from build123d import *

# Parameters (mm, degrees)
EXTRUDE_1_DEPTH             = 30
HOLE_WIZARD_M31_D           = 3.4
HOLE_WIZARD_M31_CBORE_D     = 6.5
HOLE_WIZARD_M31_CBORE_DEPTH = 3


with BuildPart() as part:
    # Эскиз1 → Бобышка-Вытянуть1 (new body)
    with BuildSketch(Plane.XY):
        Polygon((-3, 0), (-11, 0), (-11, 8), (11, 8), (11, 0), (3, 0), (3, 3), (-3, 3), align=None)
    extrude(amount=EXTRUDE_1_DEPTH)

    # Цековка для винта с внутренним шестигранником M31 (through all)
    with Locations(Plane(origin=(0, 8, 0), x_dir=(1, 0, 0), z_dir=(0, 1, 0))):
        with Locations((-7, -4), (7, -4), (7, -26), (-7, -26)):
            CounterBoreHole(HOLE_WIZARD_M31_D / 2, HOLE_WIZARD_M31_CBORE_D / 2, HOLE_WIZARD_M31_CBORE_DEPTH)


solid = part.part
Can you work these out from the model? Positions are in its coordinate system, mm. A direction names the side the tool comes from. Round coordinates to 2 decimals unless told otherwise and drop trailing zeros. Write each loop counter-clockwise with the first axis right and the second up, starting at its lowest first coordinate (ties: lowest second). Pieces come first, ordered by that corner, then holes. Notation, with made-up numbers: M 52,55 L 60,55 A32 cw 60,88 Z; hole C -6,31.25 d10. An arc over 180 degrees is marked long. Use a Markdown table: item, result.
Item 1: If I drill on line 1 along X through (y, z) = (2.45, 26); line 2 along X through (y, z) = (6.5, 26); line 3 along Z through (x, y) = (-7, 3.15), over which ranges is the centre line in solid material (lowest first)? Write a range as [from, to].
Found:
| item | result |
|---|---|
| line 1 | x = [-11, -8.7], [-5.3, -3], [3, 5.3], [8.7, 11] |
| line 2 | x = [-11, -10.25], [-3.75, 3.75], [10.25, 11] |
| line 3 | z = [0, 2.3], [5.7, 24.3], [27.7, 30] |
Item 2: I want a section at D-D (z = 19). List the corners of the cut face in (x, y) for me, and give its area (3 significant figures).
Found:
| item | result |
|---|---|
| outline | M -11,0 L -3,0 L -3,3 L 3,3 L 3,0 L 11,0 L 11,8 L -11,8 Z |
| area | 158 mm2 |
Item 3: I want a section at B-B (x = 7). List the corners of the cut face in (y, z) for me.
Found:
| item | result |
|---|---|
| outline | M 0,0 L 8,0 L 8,0.75 L 5,0.75 L 5,2.3 L 0,2.3 Z; M 0,5.7 L 5,5.7 L 5,7.25 L 8,7.25 L 8,22.75 L 5,22.75 L 5,24.3 L 0,24.3 Z; M 0,27.7 L 5,27.7 L 5,29.25 L 8,29.25 L 8,30 L 0,30 Z |
Item 4: We'd pull the mould along Z, two halves only. Please class faces 1 (the face through (3, 1, 15)), 2 (the face through (0, 4, 0)), 3 (the face through (-10.247, 6.521, 3.857)): released by +Z, released by -Z, zero draft, split by the parting line, or undercut.
Found:
| item | result |
|---|---|
| face 1 | zero draft |
| face 2 | released by -Z |
| face 3 | undercut |
Item 5: I want a section at C-C (y = 7). List the corners of the cut face in (x, z) for me.
Found:
| item | result |
|---|---|
| outline | M -11,0 L 11,0 L 11,30 L -11,30 Z; hole C -7,4 d6.5; hole C -7,26 d6.5; hole C 7,4 d6.5; hole C 7,26 d6.5 |
Item 6: I want a section at A-A (z = 26). List the corners of the cut face in (x, y) for me.
Found:
| item | result |
|---|---|
| outline | M -11,0 L -8.7,0 L -8.7,5 L -10.25,5 L -10.25,8 L -11,8 Z; M -5.3,0 L -3,0 L -3,3 L 3,3 L 3,0 L 5.3,0 L 5.3,5 L 3.75,5 L 3.75,8 L -3.75,8 L -3.75,5 L -5.3,5 Z; M 8.7,0 L 11,0 L 11,8 L 10.25,8 L 10.25,5 L 8.7,5 Z |
Item 7: Which directions (+Z, -Z, +X, -X, +Y, -Y) give clear straight access to the entire face, cutting with the end or side of a thin tool? Please do faces 4 (the face through (8.4, 5, 27.4)), 5 (the face through (0, 8, 15)), 6 (the face through (-3, 2, 15)).
Found:
| item | result |
|---|---|
| face 4 | +Y |
| face 5 | +Z, -Z, +X, -X, +Y |
| face 6 | +Z, -Z, -Y |
Item 8: For pin 1 Ø5 at (x, z) = (7.5, 3) entering from +Y; pin 2 Ø2 at (x, z) = (-7, 4) entering from +Y; pin 3 Ø3 at (x, z) = (-1, 19.5) entering from -Y; pin 4 Ø3 at (x, z) = (7.5, 25) entering from +Y, each with a flat end and sliding along its axis, tell me the tip position at first contact or that it passes through.
Found:
| item | result |
|---|---|
| pin 1 | stops at y = 8 |
| pin 2 | passes through |
| pin 3 | stops at y = 3 |
| pin 4 | stops at y = 5 |
